Design review of the part built by this model. Coordinates are the model's own, in mm. A direction names the side the tool comes from. Round coordinates to 2 decimals unless told otherwise and drop trailing zeros. Loops run counter-clockwise (first coordinate to the right, second up) from the corner with the lowest first, then second, coordinate; pieces in that order, holes last. Notation, with made-up numbers: (-38.5, 50) - (-22.5, 50) arc R25 cw to (-22.5, 67) - close; hole circle Ø2 at (33, 87). An arc over 180 degrees is marked (long way). Use one line per item in the form item = value. Start each with the question number.
(1) Machinability: for faces 1 (the flat face through (5, 0, -10)), 2 (the cylindrical face through (2.5, 0.1, -7.5)), 3 (the cylindrical face through (-7.5, -0.1, 64.1)), which of the approach directions +Z, -Z, +X, -X, +Y, -Y give a long, thin tool a straight path to every point of the face, cutting with its end or side? Answer none if there is none.
(2) We need section C-C, the plane x = 2.75. Write out the cut boundary in (y, z), then the cut area to 3 significant figures.
(3) Wall thickness on probe 1 along Y at (x, z) = (-9.75, 116); probe 2 along X at (y, z) = (-1.15, 115.5); probe 3 along Z at (x, y) = (-3, -0.3): over which ranges is each line inside the solid? List them lowest first. Write a range as [from, to].
(4) We need section B-B, the plane z = 59.5. Write out the cut boundary in (x, y).
(5) For pin 1 (1.5 mm diameter, centred on x = -2.5, y = 0.5, fed in from -Z), flat-tipped, find the tip position at first contact; note if it passes through.
(6) We need section A-A, the plane y = 0. Write out the cut boundary in (x, z), then the cut area to 3 significant figures.
from build123d import *

# Parameters (mm, degrees)
ESQUISSE1_R        = 2.5
R_VOLUTION1_ANGLE  = 90
ESQUISSE2_R        = 2.5
BOSS_EXTRU_1_DEPTH = 130
ESQUISSE3_R        = 2.5
BOSS_EXTRU_2_DEPTH = 5


with BuildPart() as part:
    # Esquisse1 → Révolution1 (revolve)
    with BuildSketch(Plane.XY):
        with Locations((-10, 0)):
            Circle(ESQUISSE1_R)
    revolve(axis=Axis((0, 7.956307344, 0), (0, -1, 0)), revolution_arc=R_VOLUTION1_ANGLE)

    # Esquisse2 → Boss.-Extru.1 (add)
    with BuildSketch(Plane.XY):
        with Locations(Location((-10, 0, 0), (0, 0, 180))):
            Circle(ESQUISSE2_R)
    extrude(amount=BOSS_EXTRU_1_DEPTH)

    # Esquisse3 → Boss.-Extru.2 (add)
    with BuildSketch(Plane(origin=(0, 0, 0), x_dir=(0, 0, -1), z_dir=(1, 0, 0))):
        with Locations((10, 0)):
            Circle(ESQUISSE3_R)
    extrude(amount=BOSS_EXTRU_2_DEPTH)


solid = part.part
Data:
q1.face_1 = +Z, -Z, +X, +Y, -Y
q1.face_2 = +X
q1.face_3 = +Z
q2.outline = circle Ø5 at (0, -10)
q2.area = 19.6 mm^2
q3.probe_1 = [-2.49, 2.49]
q3.probe_2 = [-12.22, -7.78]
q3.probe_3 = [-12.12, -6.89]
q4.outline = circle Ø5 at (-10, 0)
q5.pin_1 = -12.36
q6.outline = (-12.5, 0) arc R12.5 ccw to (0, -12.5) - (5, -12.5) - (5, -7.5) - (0, -7.5) arc R7.5 cw to (-7.5, 0) - (-7.5, 130) - (-12.5, 130) - close
q6.area = 754 mm^2
